Build history of the part. All positions in model axes, mm. Round coordinates to 2 decimals unless told otherwise and drop trailing zeros. Loops run counter-clockwise (first coordinate to the right, second up) from the corner with the lowest first, then second, coordinate; pieces in that order, holes last. Notation, with made-up numbers: M 30.5,-7 L 53.5,-7 A24 cw 53.5,27 Z; hole C 55,4 d1. An arc over 180 degrees is marked long. Use one line per item in the form item = value. Start each with the question number.
```python
from build123d import *

# Parameters (mm, degrees)
SKETCH1_R           = 5
SKETCH1_R_2         = 2.1
BOSS_EXTRUDE1_DEPTH = 3
FILLET1_R           = 5


with BuildPart() as part:
    # Sketch1 → Boss-Extrude1 (new body)
    # profile 1 of 3: a face of its own
    with BuildSketch(Plane(origin=(0, 0, 0), x_dir=(1, 0, 0), z_dir=(0, 1, 0))):
        with BuildLine():
            Line((0, 14), (0, -14))
            ThreePointArc((0, -14), (10.659672329, -20.591511651), (18.703056171, -30.202995218))
            ThreePointArc((18.703056171, -30.202995218), (20.412961628, -23.367686313), (27.260231116, -25.029048724))
            ThreePointArc((27.260231116, -25.029048724), (20.185963894, 0), (27.260231116, 25.029048724))
            ThreePointArc((27.260231116, 25.029048724), (20.412961628, 23.367686313), (18.703056171, 30.202995218))
            ThreePointArc((18.703056171, 30.202995218), (10.659672329, 20.591511651), (0, 14))
        make_face()
    # profile 2 of 3: a face of its own
    with BuildSketch(Plane(origin=(0, 0, 0), x_dir=(1, 0, 0), z_dir=(0, 1, 0))):
        with Locations((23, -27.646381495)):
            Circle(SKETCH1_R)
        with Locations(Location((23, -27.646381495, 0), (0, 0, 270))):
            Circle(SKETCH1_R_2, mode=Mode.SUBTRACT)
    # profile 3 of 3: a face of its own
    with BuildSketch(Plane(origin=(0, 0, 0), x_dir=(1, 0, 0), z_dir=(0, 1, 0))):
        with Locations((23, 27.646381495)):
            Circle(SKETCH1_R)
        with Locations(Location((23, 27.646381495, 0), (0, 0, 270))):
            Circle(SKETCH1_R_2, mode=Mode.SUBTRACT)
    extrude(amount=BOSS_EXTRUDE1_DEPTH)

    # Fillet1
    fillet1_edges = [part.edges().sort_by_distance(p)[0] for p in [
        (0, 1.5, 14),
        (0, 1.5, -14),
    ]]
    fillet(fillet1_edges, radius=FILLET1_R)


solid = part.part
```
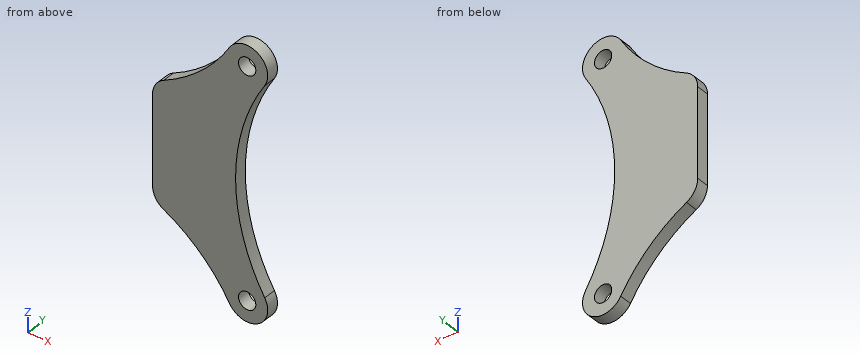
Q1. Saw through at C-C (z = -3). Give the cut face in (x, y), and give its area (3 significant figures).
Q2. Saw through at A-A (x = 22.25). Give the cut face in (y, z).
Q3. Saw through at B-B (y = 1.95). Give the cut face in (x, z), and give its area (3 significant figures).
Q4. Saw through at D-D (x = 7). Give the cut face in (y, z), and give its area (3 significant figures).
Q5. Wall check: probe 1 along X at (y, z) = (2.35, -26); probe 2 along Z at (x, y) = (25.25, 0.45); probe 3 along X at (y, z) = (2.2, 0.5). Give the ranges that are in metal, low to high.
Filled in:
q1.outline = M 0,0 L 20.28,0 L 20.28,3 L 0,3 Z
q1.area = 60.8 mm²
q2.outline = M 0,-32.59 L 3,-32.59 L 3,-29.61 L 0,-29.61 Z; M 0,-25.68 L 3,-25.68 L 3,-13.9 L 0,-13.9 Z; M 0,13.9 L 3,13.9 L 3,25.68 L 0,25.68 Z; M 0,29.61 L 3,29.61 L 3,32.59 L 0,32.59 Z
q3.outline = M 0,-10.8 A5 ccw 2.73,-15.26 A39.31 cw 18.7,-30.2 A5 ccw long 27.26,-25.03 A47.81 cw 27.26,25.03 A5 ccw long 18.7,30.2 A39.31 cw 2.73,15.26 A5 ccw 0,10.8 Z; hole C 23,-27.65 d4.2; hole C 23,27.65 d4.2
q3.area = 1,040 mm²
q4.outline = M 0,-17.78 L 3,-17.78 L 3,17.78 L 0,17.78 Z
q4.area = 107 mm²
q5.probe_1 = 15.82 to 21.7, 24.3 to 27.72
q5.probe_2 = -32.11 to -21.42, 21.42 to 32.11
q5.probe_3 = 0 to 20.19
